Read the model definition and answer for the solid it produces. Units are mm, in the model's axes. A direction names the side the tool comes from. Give positions to 0.01 mm unless a question says otherwise; leave off trailing zeros. Write each loop counter-clockwise with the first axis right and the second up, starting at its lowest first coordinate (ties: lowest second). Pieces come first, ordered by that corner, then holes. Notation, with made-up numbers: M 33.5,29 L 53.5,29 A24 ccw 53.5,59 Z; hole C -34,79 d6. An arc over 180 degrees is marked long. Write each question's results on one line, items separated by ' | '. Start each with the question number.
```python
from build123d import *

# Parameters (mm, degrees)
SKETCH_2_R          = 1.6
EXTRUDE_1_DEPTH     = 2
SKETCH_4_W          = 8.5
SKETCH_4_H          = 8
CUT_EXTRUDE_1_DEPTH = 3
SKETCH_6_R          = 1.6
CUT_EXTRUDE_2_DEPTH = 10
FILLET_1_R          = 2
FILLET_2_R          = 2


with BuildPart() as part:
    # 草图2 → 凸台-拉伸1 (new body)
    with BuildSketch(Plane.XY):
        with BuildLine():
            Line((-162.154590294, 76.5), (-162.154590294, 66.5))
            ThreePointArc((-162.154590294, 66.5), (-143.702317509, 21.952272785), (-99.154590294, 3.5))
            Line((-99.154590294, 3.5), (-88, 3.5))
            Line((-88, 3.5), (-88, -11.5))
            Line((-88, -11.5), (-99.154590294, -11.5))
            ThreePointArc((-99.154590294, -11.5), (-154.308919227, 11.345671067), (-177.154590294, 66.5))
            Line((-177.154590294, 66.5), (-177.154590294, 76.5))
            Line((-177.154590294, 76.5), (-162.154590294, 76.5))
        make_face()
        with Locations((-91.754590294, 1)):
            Circle(SKETCH_2_R, mode=Mode.SUBTRACT)
        with Locations((-99.154590294, 1)):
            Circle(SKETCH_2_R, mode=Mode.SUBTRACT)
        with Locations((-106.910050218, 1.460759219)):
            Circle(SKETCH_2_R, mode=Mode.SUBTRACT)
        with Locations((-114.556398703, 2.836554462)):
            Circle(SKETCH_2_R, mode=Mode.SUBTRACT)
        with Locations((-121.986059394, 5.108029688)):
            Circle(SKETCH_2_R, mode=Mode.SUBTRACT)
        with Locations((-129.094504517, 8.243227549)):
            Circle(SKETCH_2_R, mode=Mode.SUBTRACT)
        with Locations((-135.781725472, 12.198038998)):
            Circle(SKETCH_2_R, mode=Mode.SUBTRACT)
        with Locations((-141.953639856, 16.916823855)):
            Circle(SKETCH_2_R, mode=Mode.SUBTRACT)
        with Locations((-147.523415105, 22.333193613)):
            Circle(SKETCH_2_R, mode=Mode.SUBTRACT)
        with Locations((-152.412690143, 28.370945455)):
            Circle(SKETCH_2_R, mode=Mode.SUBTRACT)
        with Locations((-156.552677837, 34.945134346)):
            Circle(SKETCH_2_R, mode=Mode.SUBTRACT)
        with Locations((-159.885132769, 41.963268131)):
            Circle(SKETCH_2_R, mode=Mode.SUBTRACT)
        with Locations((-162.363170682, 49.326608799)):
            Circle(SKETCH_2_R, mode=Mode.SUBTRACT)
        with Locations((-163.951928103, 56.931561629)):
            Circle(SKETCH_2_R, mode=Mode.SUBTRACT)
        with Locations((-164.62905283, 64.671132664)):
            Circle(SKETCH_2_R, mode=Mode.SUBTRACT)
        with Locations((-164.654590294, 72.371090315)):
            Circle(SKETCH_2_R, mode=Mode.SUBTRACT)
    extrude(amount=EXTRUDE_1_DEPTH)

    # 草图4 → 切除-拉伸1 (cut)
    with BuildSketch(Plane.XY.offset(2)):
        with Locations((-172.904590294, 72.5)):
            Rectangle(SKETCH_4_W, SKETCH_4_H)
    extrude(amount=-CUT_EXTRUDE_1_DEPTH, mode=Mode.SUBTRACT)

    # 草图6 → 切除-拉伸2 (cut)
    with BuildSketch(Plane.XY.offset(2)):
        with Locations((-170.287955794, 46.10283567)):
            Circle(SKETCH_6_R)
        with Locations((-159.021847878, 23.00389133)):
            Circle(SKETCH_6_R)
        with Locations((-114.540055415, -5.882922454)):
            Circle(SKETCH_6_R)
        with Locations((-93.154590294, -7.5)):
            Circle(SKETCH_6_R)
    extrude(amount=-CUT_EXTRUDE_2_DEPTH, mode=Mode.SUBTRACT)

    # 圆角1
    fillet_1_edges = [part.edges().sort_by_distance(p)[0] for p in [
        (-168.654590294, 68.5, 1),
    ]]
    fillet(fillet_1_edges, radius=FILLET_1_R)

    # 圆角2
    fillet_2_edges = [part.edges().sort_by_distance(p)[0] for p in [
        (-168.654590294, 76.5, 1),
        (-162.154590294, 76.5, 1),
        (-88, 3.5, 1),
        (-88, -11.5, 1),
        (-177.154590294, 68.5, 1),
    ]]
    fillet(fillet_2_edges, radius=FILLET_2_R - 0.0001)  # a hair under: the kernel refuses the full size


solid = part.part
```
Item 1: Section A-A, the plane x = -121.5 is taken. Determine the outline of the cut face in (y, z).
Item 2: For faces 1 (the flat face through (-173, 68.5, 1)), 2 (the cylindrical face through (-149.122, 22.404, 0.986)), 3 (the flat face through (-95, 3.5, 1)), determine the directions among +Z, -Z, +X, -X, +Y, -Y from which every point of the face is accessible in a straight line to the end or side of a thin tool.
Item 3: Section C-C, the plane x = -148 is taken. Determine the outline of the cut face in (y, z).
Item 4: Section B-B, the plane z = 0.8 is taken. Give the number of separate pieces and of enclosed holes in the cut face, then the cut area to 3 significant figures.
Item 5: Straight lines are drawn through the part: line 1 (Y direction, x = -166, z = 1.5); line 2 (Y direction, x = -115, z = 1.3); line 3 (Y direction, x = -156, z = 1.7). For each, find the intervals that lie inside material, in ascending order.
Item 6: Determine the mould class of faces 4 (the cylindrical face through (-90.23, 1.48, 0.99)), 5 (the cylindrical face through (-88.6, -10.93, 1.01)), 6 (the flat face through (-142, 20, 0)) for opening direction Y: +Y half, -Y half, draft (parallel to the pull), parting line (faces both ways), or undercut.
Item 7: Given P1, Ø1, axis at x = -173, z = 1.5, coming from the +Y side; P2, Ø1, axis at x = -96.5, z = 1, coming from the +Y side; P3, Ø1, axis at x = -149, z = 1, coming from the +Y side, each flat-ended and moving along its own axis, determine where each tip first touches the part or whether it passes through.
Worked out:
1) outline: M -8.23,0 L 3.58,0 L 3.58,2 L -8.23,2 Z; M 6.63,0 L 7.6,0 L 7.6,2 L 6.63,2 Z
2) face 1: +Z, -Z, -X, +Y | face 2: +Z, -Z | face 3: +Z, -Z, +X, +Y
3) outline: M 5.69,0 L 20.81,0 L 20.81,2 L 5.69,2 Z; M 23.86,0 L 26.71,0 L 26.71,2 L 23.86,2 Z
4) separate pieces: 1 | enclosed holes: 20 | area: 1,750 mm²
5) line 1: y = 26.3 to 63.85, 65.5 to 71.51, 73.24 to 76.5 | line 2: y = -9.87 to -7.42, -4.35 to 1.3, 4.37 to 5.53 | line 3: y = 13.09 to 33.44, 36.45 to 39.34
6) face 4: undercut | face 5: -Y half | face 6: draft
7) P1: stops at y = 68.5 | P2: stops at y = 3.5 | P3: stops at y = 28.63
